Source: CAD feature listing. Evaluate the final solid. Frame: model axes, mm. A direction names the side the tool comes from. Give positions to 0.01 mm unless a question says otherwise; leave off trailing zeros. Loops run counter-clockwise (first coordinate to the right, second up) from the corner with the lowest first, then second, coordinate; pieces in that order, holes last. Notation, with made-up numbers: M 74,69 L 129,69 A18 cw 129,83 Z; hole C 39,-39 d8. An arc over 180 degrees is marked long. Answer in a Markdown table with one row per item.
```python
from build123d import *

# Parameters (mm, degrees)
SKETCH1_W           = 72
SKETCH1_H           = 57
BOSS_EXTRUDE1_DEPTH = 5
BOSS_EXTRUDE2_DEPTH = 12
SKETCH5_R           = 2.25
CUT_EXTRUDE2_DEPTH  = 64.790673299
SKETCH4_R           = 8
CUT_EXTRUDE1_DEPTH  = 64.120915709
SKETCH6_R           = 2.25
CUT_EXTRUDE3_DEPTH  = 64.120915709
SKETCH7_R           = 2.25
CUT_EXTRUDE4_DEPTH  = 64.120915709
SKETCH8_R           = 1.75
BOSS_EXTRUDE3_DEPTH = 3
SKETCH9_W           = 12
SKETCH9_H           = 10.25
BOSS_EXTRUDE4_DEPTH = 8


with BuildPart() as part:
    # Sketch1 → Boss-Extrude1 (new body)
    with BuildSketch(Plane.XY):
        with Locations((20, 0)):
            Rectangle(SKETCH1_W, SKETCH1_H)
    extrude(amount=BOSS_EXTRUDE1_DEPTH)

    # Sketch3 → Boss-Extrude2 (add)
    with BuildSketch(Plane(origin=(-16, 0, 0), x_dir=(0, 0, -1), z_dir=(1, 0, 0))):
        with BuildLine():
            Line((-5, 28.5), (-11, 28.5))
            Line((-11, 28.5), (-11, 20.5))
            ThreePointArc((-11, 20.5), (-7, 16.5), (-11, 12.5))
            Line((-11, 12.5), (-11, 4.5))
            Line((-11, 4.5), (-5, 4.5))
            Line((-5, 4.5), (-5, 28.5))
        make_face()
    boss_extrude2 = extrude(amount=BOSS_EXTRUDE2_DEPTH)

    # Sketch5 → Cut-Extrude2 (cut, through all)
    with BuildSketch(Plane.XY.offset(11)):
        with Locations((-10, 24.5)):
            Circle(SKETCH5_R)
        with Locations((-10, 8.5)):
            Circle(SKETCH5_R)
    cut_extrude2 = extrude(amount=-CUT_EXTRUDE2_DEPTH, mode=Mode.SUBTRACT)

    # Mirror1: Boss-Extrude2, Cut-Extrude2 across plane
    add(boss_extrude2.mirror(Plane(origin=(0, 0, 0), x_dir=(0, 0, 1), z_dir=(1, 0, 0))))
    add(cut_extrude2.mirror(Plane(origin=(0, 0, 0), x_dir=(0, 0, 1), z_dir=(1, 0, 0))), mode=Mode.SUBTRACT)

    # Sketch4 → Cut-Extrude1 (cut, through all)
    with BuildSketch(Plane.XY.offset(5)):
        with Locations((35, -6.5)):
            Circle(SKETCH4_R)
    extrude(amount=-CUT_EXTRUDE1_DEPTH, mode=Mode.SUBTRACT)

    # Sketch6 → Cut-Extrude3 (cut, through all)
    with BuildSketch(Plane.XY.offset(5)):
        with Locations((-11, -22.5)):
            Circle(SKETCH6_R)
        with Locations((7, -22.5)):
            Circle(SKETCH6_R)
    extrude(amount=-CUT_EXTRUDE3_DEPTH, mode=Mode.SUBTRACT)

    # Sketch7 → Cut-Extrude4 (cut, through all)
    with BuildSketch(Plane.XY.offset(5)):
        with Locations((46, 13.5)):
            Circle(SKETCH7_R)
        with Locations((24, 13.5)):
            Circle(SKETCH7_R)
    extrude(amount=-CUT_EXTRUDE4_DEPTH, mode=Mode.SUBTRACT)

    # Sketch8 → Boss-Extrude3 (add)
    with BuildSketch(Plane(origin=(0, 0, 0), x_dir=(-1, 0, 0), z_dir=(0, 0, -1))):
        Polygon((16, 39), (16, 45.5), (4, 45.5), (4, 39), (4, 28.5), (16, 28.5), align=None)
        with Locations((10, 42.25)):
            Circle(SKETCH8_R, mode=Mode.SUBTRACT)
    extrude(amount=-BOSS_EXTRUDE3_DEPTH)

    # Sketch9 → Boss-Extrude4 (add)
    with BuildSketch(Plane.XY.offset(3)):
        with Locations((-10, 33.625)):
            Rectangle(SKETCH9_W, SKETCH9_H)
    extrude(amount=BOSS_EXTRUDE4_DEPTH)


solid = part.part
```
1) Section B-B, the plane x = 24. Return loops of the section in (y, z).
Reply:
| item | result |
|---|---|
| outline | M -28.5,0 L 11.25,0 L 11.25,5 L -28.5,5 Z; M 15.75,0 L 28.5,0 L 28.5,5 L 15.75,5 Z |
2) Section C-C, the plane y = 42.25. Return loops of the section in (x, z), then the cut area to 3 significant figures.
Reply:
| item | result |
|---|---|
| outline | M -16,0 L -11.75,0 L -11.75,3 L -16,3 Z; M -8.25,0 L -4,0 L -4,3 L -8.25,3 Z |
| area | 25.5 mm² |
3) Material intervals for L1, parallel to Y at x = 10, z = 5.25; L2, parallel to Y at x = -10, z = 5.25; L3, parallel to X at y = 19.5, z = 7.25, sorted ascending.
Reply:
| item | result |
|---|---|
| L1 | y = 4.5 to 6.25, 10.75 to 22.25, 26.75 to 28.5 |
| L2 | y = 4.5 to 6.25, 10.75 to 22.25, 26.75 to 38.75 |
| L3 | x = -16 to -4, 4 to 16 |
4) Section D-D, the plane x = -6. Return loops of the section in (y, z), then the cut area to 3 significant figures.
Reply:
| item | result |
|---|---|
| outline | M -28.5,0 L 45.5,0 L 45.5,3 L 38.75,3 L 38.75,11 L 20.5,11 A4 cw 12.5,11 L 4.5,11 L 4.5,5 L -28.5,5 Z |
| area | 537 mm² |
5) Set-up query: faces 1 (the cylindrical face through (26.146, 14.176, 2.535)), 2 (the flat face through (19, 28.5, 3)), 3 (the flat face through (16, 16.7, 6.7)), 4 (the flat face through (-9, 44, 3)). Return all of +Z, -Z, +X, -X, +Y, -Y with unobstructed straight access to the full face (end or side cutting, diameter ignored); none if empty.
Reply:
| item | result |
|---|---|
| face 1 | +Z, -Z |
| face 2 | +Z, -Z, +X, +Y |
| face 3 | +Z, +X, +Y, -Y |
| face 4 | +Z, +X, -X, +Y |
6) Section A-A, the plane y = 8.5. Return loops of the section in (x, z), then the cut area to 3 significant figures.
Reply:
| item | result |
|---|---|
| outline | M -16,0 L -12.25,0 L -12.25,11 L -16,11 Z; M -7.75,0 L 7.75,0 L 7.75,11 L 4,11 L 4,5 L -4,5 L -4,11 L -7.75,11 Z; M 12.25,0 L 56,0 L 56,5 L 16,5 L 16,11 L 12.25,11 Z |
| area | 405 mm² |
7) Pull-direction query (X, two-part tool) for faces 5 (the flat face through (-16, 8, 4)), 6 (the cylindrical face through (10.488, 22.304, 5.577)), 7 (the flat face through (-10, 38.75, 7)); classes: released by +X, released by -X, zero draft, split by the parting line, or undercut.
Reply:
| item | result |
|---|---|
| face 5 | released by -X |
| face 6 | undercut |
| face 7 | zero draft |
8) Pin query (flat end, axial travel): pin 1 Ø12 at (x, y) = (8.5, -4) entering from -Z; pin 2 Ø17 at (x, y) = (13, -7.5) entering from +Z; pin 3 Ø5.5 at (x, z) = (15, 5.5) entering from +Y; pin 4 Ø5 at (y, z) = (33, 9.5) entering from +X. Return the tip coordinate at first contact, or that it passes through.
Reply:
| item | result |
|---|---|
| pin 1 | stops at z = 0 |
| pin 2 | stops at z = 5 |
| pin 3 | stops at y = 28.5 |
| pin 4 | stops at x = -4 |
